Geometry: final body of the model. Coordinates: model frame, mm. Give positions to 0.01 mm unless a question says otherwise; leave off trailing zeros. Loops run counter-clockwise (first coordinate to the right, second up) from the corner with the lowest first, then second, coordinate; pieces in that order, holes last. Notation, with made-up numbers: M -3,-12 L 5,-12 A24 cw 5,22 Z; hole C -30.75,34 d8. An arc over 180 degrees is marked long. Put each result on its own line as item: value.
```python
from build123d import *

# Parameters (mm, degrees)
F0_W        = 38
F0_H        = 26
F1_DEPTH    = 17
F2_R        = 9
F3_T1_DEPTH = 82.72135955


# Not quite as in the source:
# - a fillet or chamfer that OpenCascade refuses, or shapes differently, is made with other operations: its cross-section is extruded or revolved along the edge and cut away or added


with BuildPart() as f1:
    # F0 (on Front) → F1 (new body)
    with BuildSketch(Plane.XZ):
        with Locations((19, 13)):
            Rectangle(F0_W, F0_H)
    extrude(amount=F1_DEPTH)

    # F2
    f2_edges = [f1.edges().sort_by_distance(p)[0] for p in [
        (19, -17, 26),
    ]]
    fillet(f2_edges, radius=F2_R)

    # F3: fillet of radius 9 on 1 edges, made by hand

    # F3_s2 → F3_t1 (cut)
    with BuildSketch(Plane.YZ.offset(-22.360679775)):
        with BuildLine():
            ThreePointArc((-8, 26), (-2.2917960675, 23.05572809), (0, 17.05572809))
            Line((0, 17.05572809), (0, 26))
            Line((0, 26), (-8, 26))
        make_face()
    extrude(amount=F3_T1_DEPTH, mode=Mode.SUBTRACT)


solid = f1.part
```
Item 1: Section A-A on x = 22.5. Output: boundary loops of the cut face in (y, z).
Output values:
outline: M -17,0 L 0,0 L 0,17.06 A9 ccw -8,26 A9 ccw -17,17 Z
Item 2: Line query: probe 1 along Z at (x, y) = (4, -8.5); probe 2 along Z at (x, y) = (19.5, -15.5); probe 3 along Y at (x, z) = (32.5, 24.5). Output: solid intervals per line, ascending. Write a range as [from, to].
Output values:
probe 1: [0, 25.99]
probe 2: [0, 21.97]
probe 3: [-12.97, -3.94]
Item 3: Section B-B on y = -5.25. Output: boundary loops of the cut face in (x, z), then the cut area to 3 significant figures.
Output values:
outline: M 0,0 L 38,0 L 38,25.24 L 0,25.24 Z
area: 959 mm²
Item 4: Pin query (flat end, axial travel): pin 1 Ø1.5 at (x, z) = (20, 11) entering from +Y; pin 2 Ø1 at (x, z) = (28.5, 20.5) entering from +Y; pin 3 Ø1.5 at (x, z) = (32, 19) entering from +Y. Return the tip coordinate at first contact, or that it passes through.
Output values:
pin 1: y = 0
pin 2: y = -0.5
pin 3: y = -0.08
Item 5: Section C-C on z = 22.5. Output: boundary loops of the cut face in (x, y), then the cut area to 3 significant figures.
Output values:
outline: M 0,-15.12 L 38,-15.12 L 38,-1.83 L 0,-1.83 Z
area: 505 mm²
